The drawing under review shows one solid part. Ordinate dimensions are in mm from its lowest x, y, z. A direction names the side the tool comes from. Coordinates: 2 decimals unless noted, no trailing zeros. Order: outer loops, then holes, each group sorted by start corner. A loop starts at its lowest first (then second) coordinate and runs counter-clockwise, first axis right, second up.
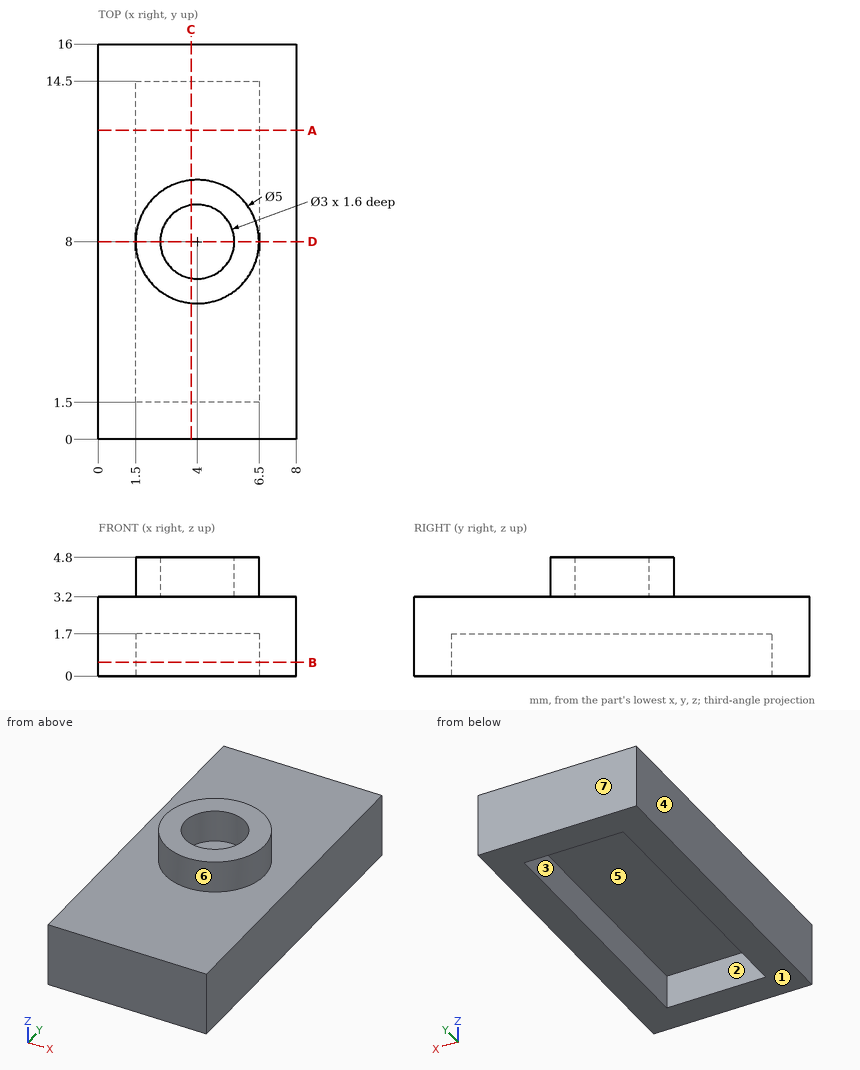
1. To check wall thickness, follow L1, parallel to Y at x = 4, z = 3.7; L2, parallel to X at y = 2, z = 0.8; L3, parallel to Y at x = 4.5, z = 0.9. State the ranges of each line that lie inside material, in increasing order.
Answer below:
L1: y = 5.5 to 6.5, 9.5 to 10.5
L2: x = 0 to 1.5, 6.5 to 8
L3: y = 0 to 1.5, 14.5 to 16
2. Clearance check with flat-ended pins moving along their axes: pin 1 Ø1 at (x, y) = (3.5, 13.5) entering from +Z; pin 2 Ø1.5 at (x, y) = (4, 8) entering from -Z. State where each tip first meets the part, or that it passes through.
Answer below:
pin 1: stops at z = 3.2
pin 2: stops at z = 1.7
3. Take a section at C-C, the plane x = 3.75. Give the boundary of the cut face in (y, z), plus the area to 3 significant figures.
Answer below:
outline: (0, 0) - (1.5, 0) - (1.5, 1.7) - (14.5, 1.7) - (14.5, 0) - (16, 0) - (16, 3.2) - (10.49, 3.2) - (10.49, 4.8) - (9.48, 4.8) - (9.48, 3.2) - (6.52, 3.2) - (6.52, 4.8) - (5.51, 4.8) - (5.51, 3.2) - (0, 3.2) - close
area: 32.3 mm2
4. Machinability: for the marked faces 5, 6 and 7, which of the approach directions +Z, -Z, +X, -X, +Y, -Y give a long, thin tool a straight path to every point of the face, cutting with its end or side? Answer none if there is none.
Answer below:
face 5: -Z
face 6: +Z
face 7: +Z, -Z, +X, -X, +Y
5. Take a section at D-D, the plane y = 8. Give the boundary of the cut face in (x, z).
Answer below:
outline: (0, 0) - (1.5, 0) - (1.5, 1.7) - (6.5, 1.7) - (6.5, 0) - (8, 0) - (8, 3.2) - (6.5, 3.2) - (6.5, 4.8) - (5.5, 4.8) - (5.5, 3.2) - (2.5, 3.2) - (2.5, 4.8) - (1.5, 4.8) - (1.5, 3.2) - (0, 3.2) - close
6. Take a section at B-B, the plane z = 0.55. Give the boundary of the cut face in (x, y).
Answer below:
outline: (0, 0) - (8, 0) - (8, 16) - (0, 16) - close; hole (1.5, 1.5) - (6.5, 1.5) - (6.5, 14.5) - (1.5, 14.5) - close
7. Take a section at A-A, the plane y = 12.5. Give the boundary of the cut face in (x, z), plus the area to 3 significant figures.
Answer below:
outline: (0, 0) - (1.5, 0) - (1.5, 1.7) - (6.5, 1.7) - (6.5, 0) - (8, 0) - (8, 3.2) - (0, 3.2) - close
area: 17.1 mm2
8. The part is to be moulded in two halves that separate along X. For the marked faces 1, 2, 3 and 4, say which applies: +X half, -X half, draft (parallel to the pull), parting line (faces both ways), or undercut.
Answer below:
face 1: draft
face 2: undercut
face 3: undercut
face 4: -X half
